Input: part model. Units: mm. Frame: model coordinates. Face numbers are marked on the shaded views. Round coordinates to 2 decimals unless told otherwise and drop trailing zeros. Loops run counter-clockwise (first coordinate to the right, second up) from the corner with the lowest first, then second, coordinate; pieces in that order, holes last. Notation, with made-up numbers: (55, 18.5) - (69, 18.5) arc R18 cw to (69, 39.5) - close; hole circle Ø2 at (6, 26.25). An arc over 180 degrees is marked (long way). One line per question, with ' | ' between items. Start each with the question number.
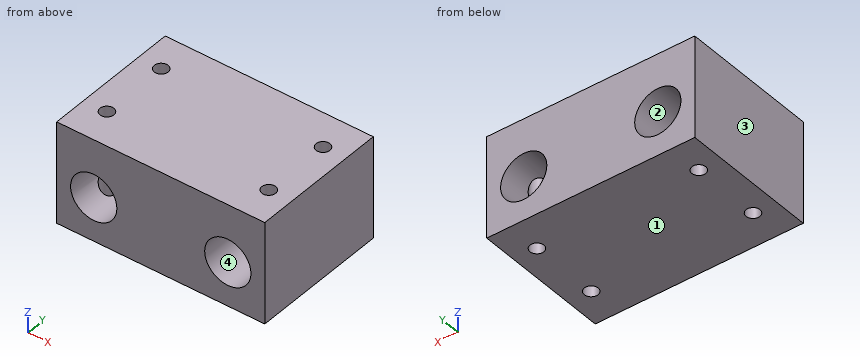
from build123d import *

# Parameters (mm, degrees)
SKETCH1_W           = 45
SKETCH1_H           = 30
BOSS_EXTRUDE2_DEPTH = 25
SKETCH4_R           = 1.5
CUT_EXTRUDE3_DEPTH  = 25
SKETCH5_R           = 5
CUT_EXTRUDE5_DEPTH  = 46.069390943
SKETCH7_W           = 45
SKETCH7_H           = 30
CUT_EXTRUDE8_DEPTH  = 3


with BuildPart() as part:
    # Sketch1 → Boss-Extrude2 (new body)
    with BuildSketch(Plane.XY):
        Rectangle(SKETCH1_W, SKETCH1_H)
    extrude(amount=BOSS_EXTRUDE2_DEPTH)

    # Sketch4 → Cut-Extrude3 (cut)
    with BuildSketch(Plane(origin=(0, 0, 0), x_dir=(-1, 0, 0), z_dir=(0, 0, -1))):
        with Locations((-17.5, 7.5)):
            Circle(SKETCH4_R)
        with Locations((17.5, 7.5)):
            Circle(SKETCH4_R)
        with Locations((-17.5, -7.5)):
            Circle(SKETCH4_R)
        with Locations((17.5, -7.5)):
            Circle(SKETCH4_R)
    extrude(amount=-CUT_EXTRUDE3_DEPTH, mode=Mode.SUBTRACT)

    # Sketch5 → Cut-Extrude5 (cut, through all)
    with BuildSketch(Plane(origin=(0, 15, 0), x_dir=(1, 0, 0), z_dir=(0, 1, 0))):
        with Locations(Location((-14.5, -12.5, 0), (0, 0, 270))):
            Circle(SKETCH5_R)
        with Locations(Location((14.5, -12.5, 0), (0, 0, 270))):
            Circle(SKETCH5_R)
    extrude(amount=-CUT_EXTRUDE5_DEPTH, mode=Mode.SUBTRACT)

    # Sketch7 → Cut-Extrude8 (cut)
    with BuildSketch(Plane(origin=(0, 0, 0), x_dir=(-1, 0, 0), z_dir=(0, 0, -1))):
        Rectangle(SKETCH7_W, SKETCH7_H)
    extrude(amount=-CUT_EXTRUDE8_DEPTH, mode=Mode.SUBTRACT)


solid = part.part
(1) Line query: line 1 along X through (y, z) = (7, 12.5); line 2 along Y through (x, z) = (17.5, 4.5); line 3 along X through (y, z) = (7.5, 7.25). Output: solid intervals per line, ascending. Write a range as from..to.
(2) Pull-direction query (X, two-part tool) for the marked faces 1, 2, 3 and 4; classes: released by +X, released by -X, zero draft, split by the parting line, or undercut.
(3) Section B-B, the plane z = 23.25. Output: boundary loops of the cut face in (x, y).
(4) Section D-D, the plane z = 15.75. Output: boundary loops of the cut face in (x, y), plus the area to 3 significant figures.
(5) Section A-A, the plane x = 14.5. Output: boundary loops of the cut face in (y, z).
(6) Pin query (flat end, axial travel): P1, Ø4, axis at x = 16, z = 14, coming from the +Y side. Return the tip coordinate at first contact, or that it passes through.
(7) Section C-C, the plane y = -4.5. Output: boundary loops of the cut face in (x, z), plus the area to 3 significant figures.
Derived:
1) line 1: x = -22.5..-19.5, -9.5..9.5, 19.5..22.5 | line 2: y = -15..-9, -6..6, 9..15 | line 3: x = -22.5..-19, -16..16, 19..22.5
2) face 1: zero draft | face 2: undercut | face 3: released by -X | face 4: undercut
3) outline: (-22.5, -15) - (22.5, -15) - (22.5, 15) - (-22.5, 15) - close; hole circle Ø3 at (-17.5, -7.5); hole circle Ø3 at (-17.5, 7.5); hole circle Ø3 at (17.5, -7.5); hole circle Ø3 at (17.5, 7.5)
4) outline: (-22.5, -15) - (-18.3, -15) - (-18.3, -8.77) arc R1.5 cw to (-18.3, -6.23) - (-18.3, 6.23) arc R1.5 cw to (-18.3, 8.77) - (-18.3, 15) - (-22.5, 15) - close; (-10.7, -15) - (10.7, -15) - (10.7, 15) - (-10.7, 15) - close; (18.3, -15) - (22.5, -15) - (22.5, 15) - (18.3, 15) - (18.3, 8.77) arc R1.5 cw to (18.3, 6.23) - (18.3, -6.23) arc R1.5 cw to (18.3, -8.77) - close | area: 889 mm²
5) outline: (-15, 3) - (15, 3) - (15, 7.5) - (-15, 7.5) - close; (-15, 17.5) - (15, 17.5) - (15, 25) - (-15, 25) - close
6) P1: passes through
7) outline: (-22.5, 3) - (22.5, 3) - (22.5, 25) - (-22.5, 25) - close; hole circle Ø10 at (-14.5, 12.5); hole circle Ø10 at (14.5, 12.5) | area: 833 mm²
